from build123d import *

# Parameters (mm, degrees)
SKETCH_W        = 105
SKETCH_H        = 120
PAD_DEPTH       = 28
SKETCH001_W     = 100.2
SKETCH001_H     = 115.2
POCKET_DEPTH    = 28.001
SKETCH002_R     = 2.5
POCKET001_DEPTH = 105.001


with BuildPart() as part:
    # Sketch → Pad (new body)
    with BuildSketch(Plane.XY):
        with Locations((0, -10)):
            Rectangle(SKETCH_W, SKETCH_H)
    extrude(amount=PAD_DEPTH)

    # Sketch001 → Pocket (cut, through all)
    with BuildSketch(Plane.XY.offset(28)):
        with Locations((0, -10)):
            Rectangle(SKETCH001_W, SKETCH001_H)
    extrude(amount=-POCKET_DEPTH, mode=Mode.SUBTRACT)

    # Sketch002 → Pocket001 (cut, through all)
    with BuildSketch(Plane(origin=(-52.5, 0, 0), x_dir=(0, -1, 0), z_dir=(-1, 0, 0))):
        with Locations((-10, 8)):
            Circle(SKETCH002_R)
        with Locations((10, 8)):
            Circle(SKETCH002_R)
        with Locations((-20, 8)):
            Circle(SKETCH002_R)
        with Locations((20, 8)):
            Circle(SKETCH002_R)
        with Locations((30, 8)):
            Circle(SKETCH002_R)
        with Locations((40, 8)):
            Circle(SKETCH002_R)
        with Locations((50, 8)):
            Circle(SKETCH002_R)
        with Locations((-30, 8)):
            Circle(SKETCH002_R)
        with Locations((0, 8)):
            Circle(SKETCH002_R)
    extrude(amount=-POCKET001_DEPTH, mode=Mode.SUBTRACT)


solid = part.part
Input: part model. Units: mm. Frame: model coordinates. A direction names the side the tool comes from. Give positions to 0.01 mm unless a question says otherwise; leave off trailing zeros. Order: outer loops, then holes, each group sorted by start corner. A loop starts at its lowest first (then second) coordinate and runs counter-clockwise, first axis right, second up. Notation, with made-up numbers: (50.25, -32) - (76.25, -32) arc R37 cw to (76.25, 5) - close; hole circle Ø4 at (-25, 50.5). An arc over 180 degrees is marked (long way). Answer as a JSON object with one key per item and string values. Group by question number.
Q1. Line query: probe 1 along X at (y, z) = (-1, 16.5); probe 2 along Y at (x, z) = (-30, 10.5); probe 3 along Z at (x, y) = (51.5, 10). Output: solid intervals per line, ascending.
Q2. First-contact query: pin 1 Ø4 at (y, z) = (-10, 8) entering from +X; pin 2 Ø6.5 at (y, z) = (0, 8) entering from +X. Flat tips, straight axial feed; report the tip coordinate or a pass-through.
Q3. Cut plane B-B, the plane x = -9. Output: boundary loops of the cut face in (y, z).
Q4. Cut plane D-D, the plane y = -61. Output: boundary loops of the cut face in (x, z).
Q5. Mould query, pull axis Y, two halves, no side actions, for faces 1 (the face through (-1, -70, 14)), 2 (the face through (0, 48, 0)), 3 (the face through (-51.32, -29.46, 5.56)). Classes: pulls with the +Y half, pulls with the -Y half, needs draft (parallel to the pull), parting line crosses it, or undercut.
Q6. Cut plane A-A, the plane y = 10. Output: boundary loops of the cut face in (x, z), then the cut area to 3 significant figures.
Q7. Set-up query: faces 4 (the face through (52.5, -11, 14)), 5 (the face through (-1, -67.6, 14)). Return all of +Z, -Z, +X, -X, +Y, -Y with unobstructed straight access to the full face (end or side cutting, diameter ignored); none if empty.
Q8. Cut plane C-C, the plane z = 14.25. Output: boundary loops of the cut face in (x, y), then the cut area to 3 significant figures.
Results:
{
 "1": {"probe 1": "-52.5 to -50.1, 50.1 to 52.5", "probe 2": "-70 to -67.6, 47.6 to 50", "probe 3": "0 to 5.5, 10.5 to 28"},
 "2": {"pin 1": "through", "pin 2": "x = 52.5"},
 "3": {"outline": "(-70, 0) - (-67.6, 0) - (-67.6, 28) - (-70, 28) - close; (47.6, 0) - (50, 0) - (50, 28) - (47.6, 28) - close"},
 "4": {"outline": "(-52.5, 0) - (-50.1, 0) - (-50.1, 28) - (-52.5, 28) - close; (50.1, 0) - (52.5, 0) - (52.5, 28) - (50.1, 28) - close"},
 "5": {"face 1": "pulls with the -Y half", "face 2": "needs draft", "face 3": "undercut"},
 "6": {"outline": "(-52.5, 0) - (-50.1, 0) - (-50.1, 5.5) - (-52.5, 5.5) - close; (-52.5, 10.5) - (-50.1, 10.5) - (-50.1, 28) - (-52.5, 28) - close; (50.1, 0) - (52.5, 0) - (52.5, 5.5) - (50.1, 5.5) - close; (50.1, 10.5) - (52.5, 10.5) - (52.5, 28) - (50.1, 28) - close", "area": "110 mm^2"},
 "7": {"face 4": "+Z, -Z, +X, +Y, -Y", "face 5": "+Z, -Z"},
 "8": {"outline": "(-52.5, -70) - (52.5, -70) - (52.5, 50) - (-52.5, 50) - close; hole (-50.1, -67.6) - (50.1, -67.6) - (50.1, 47.6) - (-50.1, 47.6) - close", "area": "1,060 mm^2"}
}
